Geometry check sheet. Reference: the model listing, model coordinates, mm. A direction names the side the tool comes from. Coordinates: 2 decimals unless noted, no trailing zeros. Write each loop counter-clockwise with the first axis right and the second up, starting at its lowest first coordinate (ties: lowest second). Pieces come first, ordered by that corner, then holes. Notation, with made-up numbers: (-14, 23.5) -> (-10, 23.5) arc R22 ccw to (-10, 50.5) -> close; hole circle Ø4 at (6.25, 21). An arc over 180 degrees is marked (long way). Answer in a Markdown table with one row per item. Add a question column.
Q1. Thickness scan on line 1 (Y direction, x = 254, z = 5.75) (3 decimals); line 2 (Y direction, x = 18, z = 29) (3 decimals); line 3 (X direction, y = 110.5, z = 21.5). Record the ranges inside material, lowest first.
Q2. Gauge pin test, flat ends, axial feed: P1, Ø2, axis at x = 183, z = 78, coming from the +Y side (3 decimals); P2, Ø4, axis at y = 80.5, z = 54.5, coming from the -X side; P3, Ø21, axis at x = 46, z = 6, coming from the -Y side. Record the tip position at first contact, or that the pin passes through.
Q3. Tool access check on faces 1 (the face through (104.766, 192.837, 9.658)), 2 (the face through (175, 10, 101.6)), 3 (the face through (175, 19.05, 60)). Record the directions out of +Z, -Z, +X, -X, +Y, -Y that give a thin tool (end or side, any length) a straight path to the whole face; none if there is none.
Q4. Section check D-D, the plane x = 113.5. Record the boundary of the cut face in (y, z) (3 decimals), and give its area (3 significant figures).
Q5. Section check A-A, the plane x = 34. Record the boundary of the cut face in (y, z) (3 decimals).
Q6. Section check C-C, the plane y = 90.5. Record the boundary of the cut face in (x, z) (3 decimals).
Q7. Release check for a two-part mould opening along X. For faces 4 (the face through (46, 231.775, 10)), 5 (the face through (365, 135, 123.825)), 6 (the face through (0, 130, 16)), 7 (the face through (25.4, 194, 10)) record: pulls with the +X half, pulls with the -X half, needs draft (parallel to the pull), parting line crosses it, or undercut.
```python
from build123d import *

# Parameters (mm, degrees)
F0_W      = 355.6
F0_H      = 263.525
F1_DEPTH  = 19.05
F2_W      = 355.6
F2_H      = 19.05
F3_DEPTH  = 82.55
F4_W      = 19.05
F4_H      = 400.05
F5_DEPTH  = 123.825
F6_R      = 7.9375
F8_DEPTH  = 25.4
F9_R      = 3.571875
F10_DEPTH = 25.4


with BuildPart() as f1:
    # F0 (on Top) → F1 (new body)
    with BuildSketch(Plane.XY):
        with Locations((177.8, 131.7625)):
            Rectangle(F0_W, F0_H)
    extrude(amount=F1_DEPTH)

    # F2 (on face) → F3 (join)
    with BuildSketch(Plane.XY.offset(19.05)):
        with Locations((177.8, 254)):
            Rectangle(F2_W, F2_H)
        with Locations((177.8, 9.525)):
            Rectangle(F2_W, F2_H)
    extrude(amount=F3_DEPTH)

    # F4 (on Top) → F5 (join)
    with BuildSketch(Plane.XY):
        with Locations((365.125, 131.7752)):
            Rectangle(F4_W, F4_H)
    extrude(amount=F5_DEPTH)

    # F6
    f6_edges = [f1.edges().sort_by_distance(p)[0] for p in [
        (374.65, 331.8002, 61.9125),
        (374.65, -68.2498, 61.9125),
    ]]
    fillet(f6_edges, radius=F6_R)

    # F7 (on face) → F8 (cut)
    with BuildSketch(Plane.XY.offset(19.05)):
        with BuildLine():
            Line((66.675, 231.775), (25.4, 231.775))
            Line((25.4, 231.775), (25.4, 155.575))
            Line((25.4, 155.575), (66.675, 155.575))
            ThreePointArc((66.675, 155.575), (104.775, 193.675), (66.675, 231.775))
        make_face()
    extrude(amount=-F8_DEPTH, mode=Mode.SUBTRACT)

    # F9 (on face) → F10 (cut)
    with BuildSketch(Plane.XY.offset(19.05)):
        with Locations((152.4, 207.9752)):
            Circle(F9_R)
        with Locations((152.4, 55.5752)):
            Circle(F9_R)
        with Locations((254, 207.9752)):
            Circle(F9_R)
        with Locations((254, 55.5752)):
            Circle(F9_R)
    extrude(amount=-F10_DEPTH, mode=Mode.SUBTRACT)


solid = f1.part
```
Calculated:
| question | item | result |
|---|---|---|
| 1 | line 1 | y = 0 to 52.003, 59.147 to 204.403, 211.547 to 263.525 |
| 1 | line 2 | y = 0 to 19.05, 244.475 to 263.525 |
| 1 | line 3 | x = 355.6 to 374.65 |
| 2 | P1 | stops at y = 263.525 |
| 2 | P2 | stops at x = 355.6 |
| 2 | P3 | stops at y = 0 |
| 3 | face 1 | +Z, -Z |
| 3 | face 2 | +Z, -X, +Y, -Y |
| 3 | face 3 | +Z, -X |
| 4 | outline | (0, 0) -> (263.525, 0) -> (263.525, 101.6) -> (244.475, 101.6) -> (244.475, 19.05) -> (19.05, 19.05) -> (19.05, 101.6) -> (0, 101.6) -> close |
| 4 | area | 8,170 mm² |
| 5 | outline | (0, 0) -> (155.575, 0) -> (155.575, 19.05) -> (19.05, 19.05) -> (19.05, 101.6) -> (0, 101.6) -> close; (231.775, 0) -> (263.525, 0) -> (263.525, 101.6) -> (244.475, 101.6) -> (244.475, 19.05) -> (231.775, 19.05) -> close |
| 6 | outline | (0, 0) -> (374.65, 0) -> (374.65, 123.825) -> (355.6, 123.825) -> (355.6, 19.05) -> (0, 19.05) -> close |
| 7 | face 4 | undercut |
| 7 | face 5 | needs draft |
| 7 | face 6 | pulls with the -X half |
| 7 | face 7 | undercut |
